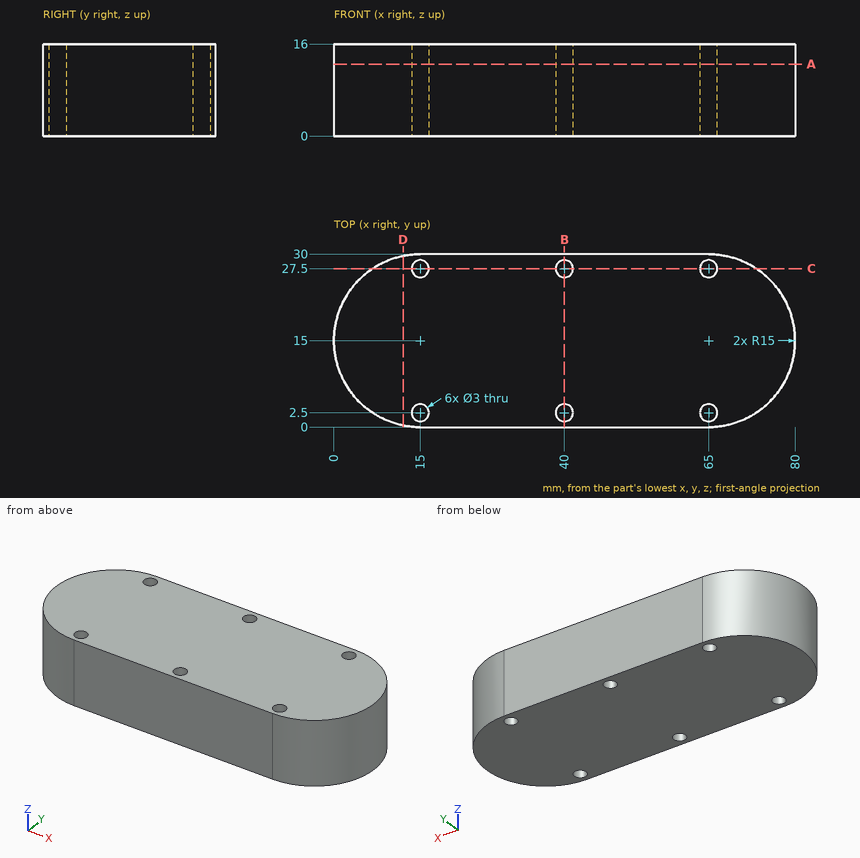
Input: dimensioned drawing with shaded views. Units: mm. Origin: part minimum x, y, z. Coordinates: 2 decimals unless noted, no trailing zeros. Loops run counter-clockwise (first coordinate to the right, second up) from the corner with the lowest first, then second, coordinate; pieces in that order, holes last. Notation, with made-up numbers: (58.25, -25) -> (80.25, -25) arc R5 cw to (80.25, -21) -> close; hole circle Ø1 at (-20, -39.5). An arc over 180 degrees is marked (long way). One line per item, written item: value. Start each with the question number.
Q1. Section query C-C, the plane y = 27.5. Return the cut outline in (x, z), and give its area (3 significant figures).
Q2. Section query D-D, the plane x = 12. Return the cut outline in (y, z).
Q3. Section query A-A, the plane z = 12.5. Return the cut outline in (x, y), and give its area (3 significant figures).
Q4. Line query: line 1 along Y through (x, z) = (40, 6.25); line 2 along X through (y, z) = (26.5, 11.25); line 3 along X through (y, z) = (28.5, 1.5). Output: solid intervals per line, ascending.
Q5. Contact query for flat-ended pins moving along their axis: P1, Ø3.5, axis at x = 65, y = 2.5, coming from the +Z side; P2, Ø1, axis at x = 67.5, z = 14, coming from the +Y side; P3, Ø1, axis at y = 6, z = 12, coming from the +X side; P4, Ø1, axis at y = 11, z = 7.5, coming from the -X side. Output: stop coordinate, or through.
Q6. Section query B-B, the plane x = 40. Return the cut outline in (y, z), and give its area (3 significant figures).
Results:
1. outline: (6.71, 0) -> (13.5, 0) -> (13.5, 16) -> (6.71, 16) -> close; (16.5, 0) -> (38.5, 0) -> (38.5, 16) -> (16.5, 16) -> close; (41.5, 0) -> (63.5, 0) -> (63.5, 16) -> (41.5, 16) -> close; (66.5, 0) -> (73.29, 0) -> (73.29, 16) -> (66.5, 16) -> close
1. area: 921 mm^2
2. outline: (0.3, 0) -> (29.7, 0) -> (29.7, 16) -> (0.3, 16) -> close
3. outline: (15, 0) -> (65, 0) arc R15 ccw to (65, 30) -> (15, 30) arc R15 ccw to start; hole circle Ø3 at (15, 2.5); hole circle Ø3 at (15, 27.5); hole circle Ø3 at (40, 2.5); hole circle Ø3 at (40, 27.5); hole circle Ø3 at (65, 2.5); hole circle Ø3 at (65, 27.5)
3. area: 2,160 mm^2
4. line 1: 0 to 1, 4 to 26, 29 to 30
4. line 2: 5.37 to 13.88, 16.12 to 38.88, 41.12 to 63.88, 66.12 to 74.63
4. line 3: 8.46 to 13.88, 16.12 to 38.88, 41.12 to 63.88, 66.12 to 71.54
5. P1: z = 16
5. P2: y = 29.87
5. P3: x = 77.36
5. P4: x = 0.41
6. outline: (0, 0) -> (1, 0) -> (1, 16) -> (0, 16) -> close; (4, 0) -> (26, 0) -> (26, 16) -> (4, 16) -> close; (29, 0) -> (30, 0) -> (30, 16) -> (29, 16) -> close
6. area: 384 mm^2
